from build123d import *

# Parameters (mm, degrees)
BASPROSKE_W             = 5
BASPROSKE_H             = 22.5
TOOTHCUT_DEPTH          = 33.210246817
TEETHCUTS_COUNT         = 16
TEETHCUTS_ANGLE         = 337.5
BORSKE_R                = 2.5
BORE_DEPTH              = 50.0000508
ENL_V_START             = -3
ESQUISSE3_R             = 10
ENL_V_MAT_EXTRU_3_DEPTH = 29.756555396
ESQUISSE8_R             = 1.5
ENL_V_MAT_EXTRU_4_DEPTH = 32.756555396


with BuildPart() as part:
    # BasProSke → Base-Revolve (revolve)
    with BuildSketch(Plane(origin=(0, 0, 0), x_dir=(1, 0, 0), z_dir=(0, 1, 0)), mode=Mode.PRIVATE) as base_revolve_sk:
        with Locations((2.5, 11.25)):
            Rectangle(BASPROSKE_W, BASPROSKE_H)
    revolve(base_revolve_sk.sketch.rotate(Axis((-10, 0, 0), (1, 0, 0)), 180), axis=Axis((-10, 0, 0), (1, 0, 0)))

    # TooCutSke → ToothCut (cut, through all)
    with BuildSketch(Plane(origin=(0, 0, 0), x_dir=(0, 0, -1), z_dir=(1, 0, 0))):
        with BuildLine():
            ThreePointArc((1.297749273, 16.824022195), (0, 16.874), (-1.297749273, 16.824022195))
            ThreePointArc((-1.297749273, 16.824022195), (-2.047921493, 19.754510488), (-3.832565589, 22.196961192))
            ThreePointArc((-3.832565589, 22.196961192), (0, 22.5254), (3.832565589, 22.196961192))
            ThreePointArc((3.832565589, 22.196961192), (2.047921493, 19.754510488), (1.297749273, 16.824022195))
        make_face()
    toothcut = extrude(amount=TOOTHCUT_DEPTH, mode=Mode.SUBTRACT)

    # TeethCuts: ToothCut ×16 about axis
    teethcuts_axis = Axis((-10, 0, 0), (1, 0, 0))
    for i in range(1, TEETHCUTS_COUNT):
        add(toothcut.rotate(teethcuts_axis, i * TEETHCUTS_ANGLE / (TEETHCUTS_COUNT - 1)), mode=Mode.SUBTRACT)

    # BorSke → Bore (cut, symmetric)
    with BuildSketch(Plane(origin=(0, 0, 0), x_dir=(0, 0, -1), z_dir=(1, 0, 0))):
        with Locations(Location((0, 0, 0), (0, 0, 180))):
            Circle(BORSKE_R)
    extrude(amount=BORE_DEPTH, both=True, mode=Mode.SUBTRACT)

    # Esquisse3 → Enlèv. mat.-Extru.3 (cut, through all)
    with BuildSketch(Plane(origin=(5, 0, 0), x_dir=(0, 0, -1), z_dir=(1, 0, 0)).offset(ENL_V_START)):
        Circle(ESQUISSE3_R)
    extrude(amount=-ENL_V_MAT_EXTRU_3_DEPTH, mode=Mode.SUBTRACT)

    # Esquisse8 → Enlèv. mat.-Extru.4 (cut, through all)
    with BuildSketch(Plane.ZY):
        with Locations((5.060877471, 4.836064435)):
            Circle(ESQUISSE8_R)
        with Locations((-4.836064435, 5.060877471)):
            Circle(ESQUISSE8_R)
        with Locations((4.836064435, -5.060877471)):
            Circle(ESQUISSE8_R)
        with Locations((-5.060877471, -4.836064435)):
            Circle(ESQUISSE8_R)
    extrude(amount=-ENL_V_MAT_EXTRU_4_DEPTH, mode=Mode.SUBTRACT)


solid = part.part
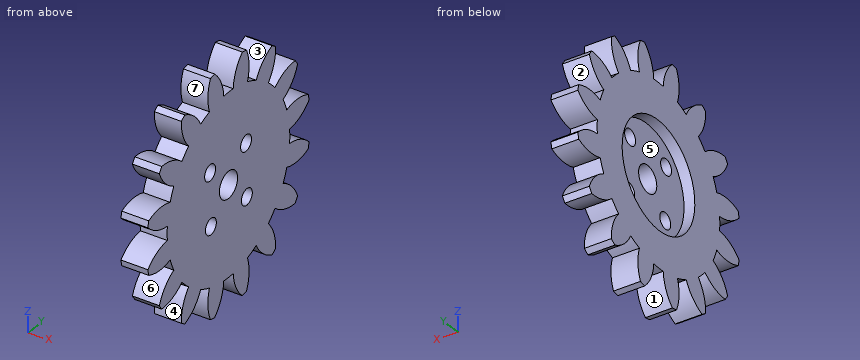
The listing builds one solid part. Answer for the finished solid, in the listing's coordinates (mm). Face numbers are marked on the shaded views. A direction names the side the tool comes from. Give positions to 0.01 mm unless a question says otherwise; leave off trailing zeros. Order: outer loops, then holes, each group sorted by start corner. A loop starts at its lowest first (then second) coordinate and runs counter-clockwise, first axis right, second up. Notation, with made-up numbers: (-7.75, 35) -> (0.25, 35) arc R32 ccw to (0.25, 74) -> close; hole circle Ø5 at (38.25, 38). An arc over 180 degrees is marked (long way). Put each result on its own line as item: value.
Item 1: A cutting plane is placed at D-D on y = 11.5. Give the vertices of the cut face in (x, z).
Established:
outline: (0, -18.82) -> (5, -18.82) -> (5, -13.47) -> (0, -13.47) -> close; (0, -12.35) -> (5, -12.35) -> (5, 12.35) -> (0, 12.35) -> close; (0, 13.47) -> (5, 13.47) -> (5, 18.82) -> (0, 18.82) -> close
Item 2: Given P1, Ø1.8, axis at y = -5.06, z = 4.84, coming from the -X side; P2, Ø1.5, axis at x = 2, y = -15.5, coming from the +Z side; P3, Ø1, axis at x = 1, z = 13, coming from the +Y side; P4, Ø6, axis at y = 2.5, z = 3, coming from the -X side, each flat-ended and moving along its own axis, determine where each tip first touches the part or whether it passes through.
Established:
P1: passes through
P2: stops at z = 12.77
P3: stops at y = 18.71
P4: stops at x = 2
Item 3: For a pull along Z with two mould halves and no side action, classify the marked faces 1, 2, 3 and 4 as released by +Z, released by -Z, zero draft, split by the parting line, or undercut.
Established:
face 1: released by -Z
face 2: undercut
face 3: released by +Z
face 4: undercut
Item 4: A cutting plane is placed at A-A on y = 0. Give the vertices of the cut face in (x, z).
Established:
outline: (0, -16.87) -> (5, -16.87) -> (5, -2.5) -> (2, -2.5) -> (2, -10) -> (0, -10) -> close; (0, 10) -> (2, 10) -> (2, 2.5) -> (5, 2.5) -> (5, 16.87) -> (0, 16.87) -> close
Item 5: Straight lines are drawn through the part: line 1 (Y direction, x = 1.7, z = 18.5); line 2 (X direction, y = -8, z = -5); line 3 (Y direction, x = 1.9, z = 11.5). For each, find the intervals that lie inside material, in ascending order.
Established:
line 1: y = -12.81 to -10.88, -5.68 to -1.58, 1.58 to 5.68, 10.88 to 12.81
line 2: x = 2 to 5
line 3: y = -18.82 to -13.47, -12.35 to 12.35, 13.47 to 18.82
Item 6: For the marked faces 5, 6 and 7, determine the directions among +Z, -Z, +X, -X, +Y, -Y from which every point of the face is accessible in a straight line to the end or side of a thin tool.
Established:
face 5: -X
face 6: +X, -X, -Y
face 7: +X, -X
Item 7: A cutting plane is placed at C-C on z = -17.5. Give the vertices of the cut face in (x, y), plus the area to 3 significant figures.
Established:
outline: (0, -12.97) -> (5, -12.97) -> (5, -9.49) -> (0, -9.49) -> close; (0, -5.59) -> (5, -5.59) -> (5, -1.37) -> (0, -1.37) -> close; (0, 1.37) -> (5, 1.37) -> (5, 5.59) -> (0, 5.59) -> close; (0, 9.49) -> (5, 9.49) -> (5, 12.97) -> (0, 12.97) -> close
area: 77.0 mm^2
